Build history of the part. All positions in model axes, mm. Give positions to 0.01 mm unless a question says otherwise; leave off trailing zeros. Order: outer loops, then holes, each group sorted by start corner. A loop starts at its lowest first (then second) coordinate and runs counter-clockwise, first axis right, second up. Notation, with made-up numbers: (-4, 77) - (37, 77) arc R28 cw to (37, 109) - close; hole circle Ø11 at (56, -17). An arc over 180 degrees is marked (long way). One line per item, written item: value.
```python
from build123d import *

# Parameters (mm, degrees)
F0_W     = 152.4
F0_H     = 342.9
F1_DEPTH = 4.7625
F2_W     = 25.4
F2_H     = 4.7625
F3_DEPTH = 9.525
F4_W     = 152.4
F4_H     = 4.7625
F5_DEPTH = 9.525


with BuildPart() as f1:
    # F0 (on Front) → F1 (new body)
    with BuildSketch(Plane.XZ):
        Rectangle(F0_W, F0_H)
    extrude(amount=F1_DEPTH)

    # F2 (on face) → F3 (join)
    with BuildSketch(Plane.XZ.offset(4.7625)):
        with Locations((-50.8, 169.06875)):
            Rectangle(F2_W, F2_H)
        with Locations((50.8, 169.06875)):
            Rectangle(F2_W, F2_H)
    extrude(amount=-F3_DEPTH)

    # F4 (on face) → F5 (join)
    with BuildSketch(Plane.XZ.offset(4.7625)):
        with Locations((0, -169.06875)):
            Rectangle(F4_W, F4_H)
    extrude(amount=-F5_DEPTH)


solid = f1.part
```
(1) Pin check, flat tips, straight feed: P1, Ø2, axis at x = -31.5, z = -50.5, coming from the +Y side; P2, Ø5, axis at y = 1.5, z = 169, coming from the +X side; P3, Ø5, axis at y = 3, z = 170, coming from the -X side; P4, Ø1, axis at y = 2, z = 3, coming from the +X side. Stop position of each tip, or through.
Completed:
P1: y = 0
P2: x = 76.2
P3: x = -63.5
P4: through
(2) Drill centre lines: line 1 (Z direction, x = 69.5, y = 1.5); line 2 (Y direction, x = 15, z = -77.5); line 3 (Z direction, x = -57.5, y = 1.5). Where is each one in solid material? Low to high.
Completed:
line 1: -171.45 to -166.69
line 2: -4.76 to 0
line 3: -171.45 to -166.69, 166.69 to 171.45
(3) Slice it at C-C, the plane z = 53. Give the cut face in (x, y), and give its area (3 significant figures).
Completed:
outline: (-76.2, -4.76) - (76.2, -4.76) - (76.2, 0) - (-76.2, 0) - close
area: 726 mm²
(4) Slice it at D-D, the plane x = -17.5. Give the cut face in (y, z).
Completed:
outline: (-4.76, -171.45) - (4.76, -171.45) - (4.76, -166.69) - (0, -166.69) - (0, 171.45) - (-4.76, 171.45) - close
(5) Slice it at B-B, the plane x = 42. Give the cut face in (y, z).
Completed:
outline: (-4.76, -171.45) - (4.76, -171.45) - (4.76, -166.69) - (0, -166.69) - (0, 166.69) - (4.76, 166.69) - (4.76, 171.45) - (-4.76, 171.45) - close
(6) Pull direction Z, two halves, no side cores. Call faces 1 (the face through (-1, 0, -171.45)), 2 (the face through (-1, 0, 5)), 3 (the face through (76.2, -2, -2)), 4 (the face through (-1, -2, 171.45)): +Z half, -Z half, draft (parallel to the pull), parting line (faces both ways), or undercut.
Completed:
face 1: -Z half
face 2: undercut
face 3: draft
face 4: +Z half
(7) Slice it at A-A, the plane y = 2. Give the cut face in (x, z), and give its area (3 significant figures).
Completed:
outline: (-76.2, -171.45) - (76.2, -171.45) - (76.2, -166.69) - (-76.2, -166.69) - close; (-63.5, 166.69) - (-38.1, 166.69) - (-38.1, 171.45) - (-63.5, 171.45) - close; (38.1, 166.69) - (63.5, 166.69) - (63.5, 171.45) - (38.1, 171.45) - close
area: 968 mm²
